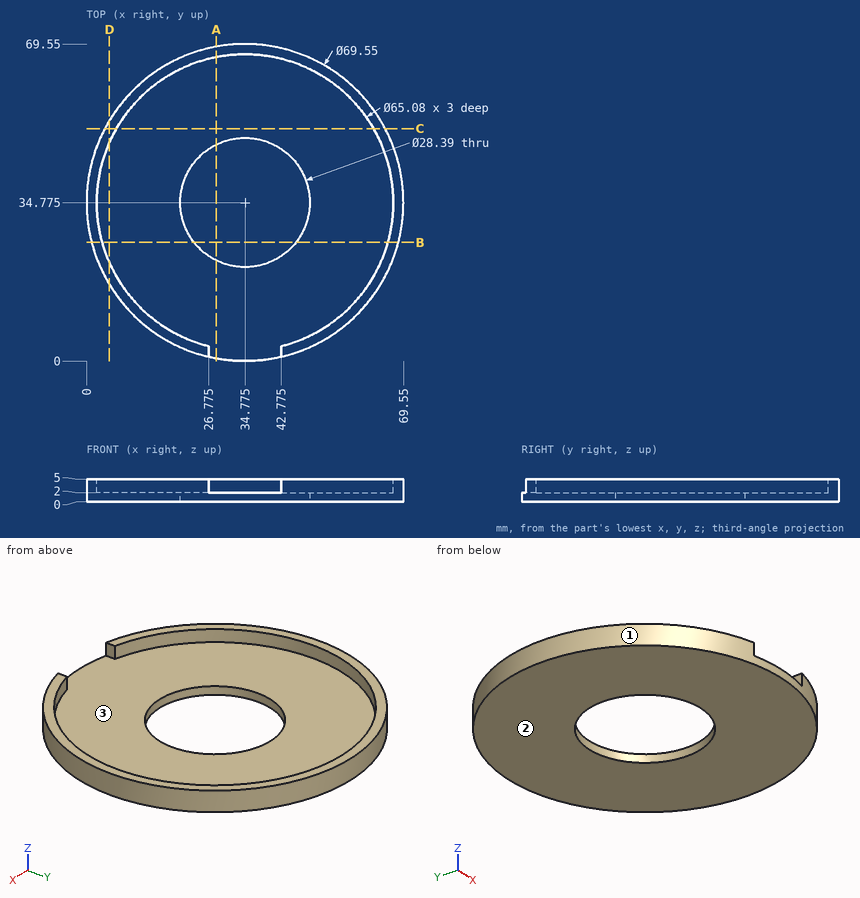
Print and shaded views of the part. All mm, measured from the part's lowest x, y and z. Round coordinates to 2 decimals unless told otherwise and drop trailing zeros. Write each loop counter-clockwise with the first axis right and the second up, starting at its lowest first coordinate (ties: lowest second). Pieces come first, ordered by that corner, then holes. Notation, with made-up numbers: M 87.25,13 L 128.25,13 A13 ccw 128.25,37 Z; hole C 77,-7 d10. An arc over 180 degrees is marked long. Use a Markdown table: item, result. Add a question column.
1. Slice it at D-D on x = 5. Give the cut face in (y, z).
2. Drill centre lines: probe 1 along Z at (x, y) = (23, 7); probe 2 along X at (y, z) = (36.5, 1.45); probe 3 along Y at (x, z) = (63.5, 3.85). Where is each one in solid material? Low to high.
3. Pull direction Y, two halves, no side cores. Call the marked faces 1, 2 and 3: released by +Y, released by -Y, zero draft, split by the parting line, or undercut.
4. Slice it at C-C on y = 51. Give the cut face in (x, z).
5. Flat gauge pins, fed straight in: P1, Ø1.8, axis at y = 2, z = 3, coming from the -X side; P2, Ø1.5, axis at y = 28, z = 0.5, coming from the +X side; P3, Ø19.5, axis at x = 31, y = 46.5, coming from the +Z side. Where does each tip first touch, or does it go through?
6. Slice it at B-B on y = 26. Give the cut face in (x, z), then the cut area to 3 significant figures.
7. Slice it at A-A on x = 28.5. Give the cut face in (y, z), then the cut area to 3 significant figures.
Reply:
| question | item | result |
|---|---|---|
| 1 | outline | M 16.81,0 L 52.74,0 L 52.74,5 L 47.9,5 L 47.9,2 L 21.65,2 L 21.65,5 L 16.81,5 Z |
| 2 | probe 1 | z = 0 to 2 |
| 2 | probe 2 | x = 0.04 to 20.69, 48.86 to 69.51 |
| 2 | probe 3 | y = 15.17 to 19.49, 50.06 to 54.38 |
| 3 | face 1 | split by the parting line |
| 3 | face 2 | zero draft |
| 3 | face 3 | undercut |
| 4 | outline | M 4.02,0 L 65.53,0 L 65.53,5 L 62.98,5 L 62.98,2 L 6.57,2 L 6.57,5 L 4.02,5 Z |
| 5 | P1 | stops at x = 20.87 |
| 5 | P2 | stops at x = 69.02 |
| 5 | P3 | stops at z = 2 |
| 6 | outline | M 1.13,0 L 23.62,0 L 23.62,2 L 3.44,2 L 3.44,5 L 1.13,5 Z; M 45.93,0 L 68.42,0 L 68.42,5 L 66.11,5 L 66.11,2 L 45.93,2 Z |
| 6 | area | 104 mm^2 |
| 7 | outline | M 0.57,0 L 22.04,0 L 22.04,2 L 0.57,2 Z; M 47.51,0 L 68.98,0 L 68.98,5 L 66.7,5 L 66.7,2 L 47.51,2 Z |
| 7 | area | 92.7 mm^2 |
